from build123d import *

# Parameters (mm, degrees)
F2_R     = 1.5
F3_DEPTH = 25
F7_R     = 4


with BuildPart() as f1:
    # F0 (on Top) → F1 (revolve)
    with BuildSketch(Plane.XY):
        Polygon((0, 5), (0, 0), (11, 0), (11, 25), (9, 25), (9, 28), (5, 28), (5, 25), (3, 25), (3, 5), align=None)
    revolve(axis=Axis((5.5, 0, 0), (1, 0, 0)))

    # F2 (on face) → F3 (cut)
    with BuildSketch(Plane(origin=(0, 0, 0), x_dir=(0, -1, 0), z_dir=(-1, 0, 0))):
        Circle(F2_R)
    extrude(amount=-F3_DEPTH, mode=Mode.SUBTRACT)

    # F5 (on Top) → F6 (revolve)
    with BuildSketch(Plane.XY):
        Polygon((3, 25), (11, 25), (11, 26), (9, 28), (5, 28), (3, 26), align=None)
    revolve(axis=Axis((0, 0, 0), (-1, 0, 0)))

    # F7
    f7_edges = [f1.edges().sort_by_distance(p)[0] for p in [
        (9, -28, 0),
        (5, -28, 0),
    ]]
    fillet(f7_edges, radius=F7_R)


solid = f1.part
For this review, take the finished solid that the model builds, in its own axes (mm). A direction names the side the tool comes from. Round coordinates to 2 decimals unless told otherwise and drop trailing zeros. Put each result on its own line as item: value.
Q1. Machinability: for faces 1 (the cylindrical face through (1.48, -1.08, -4.88)), 2 (the flat face through (0, -1.2, 1.2)), which of the approach directions +Z, -Z, +X, -X, +Y, -Y give a long, thin tool a straight path to every point of the face, cutting with its end or side? Answer none if there is none.
Check result:
face 1: -X
face 2: +Z, -Z, -X, +Y, -Y
Q2. Mouldability with a two-part tool opening along Y and no side actions: class faces 3 (the cylindrical face through (6.995, 25.865, -10.724)), 4 (the flat face through (11, -5, 0)), 5 (the cylindrical face through (5.42, 1.5, 0.07)) as pulls with the +Y half, pulls with the -Y half, needs draft (parallel to the pull), parting line crosses it, or undercut.
Check result:
face 3: parting line crosses it
face 4: needs draft
face 5: undercut
Q3. For probe 1 along Z at (x, y) = (7, 0); probe 2 along X at (y, z) = (5.5, -8.5); probe 3 along X at (y, z) = (22, 16), list the stretches that pass through material, from the lowest coordinate up. Write a range as [from, to].
Check result:
probe 1: [-28, -1.5], [1.5, 28]
probe 2: [3, 11]
probe 3: [4.26, 9.74]
Q4. Insertion check: pin 1 Ø15.5 at (y, z) = (-7, -5.5) entering from -X; pin 2 Ø10 at (y, z) = (-14, 9) entering from -X; pin 3 Ø5 at (x, y) = (2, 5) entering from -Z; pin 4 Ø5 at (x, z) = (9, -14.5) entering from +Y. Each pin has a flat end and moves straight along its axis. Give the tip position at first contact, or say it passes through.
Check result:
pin 1: x = 0
pin 2: x = 3
pin 3: z = -26.96
pin 4: y = 25.14
